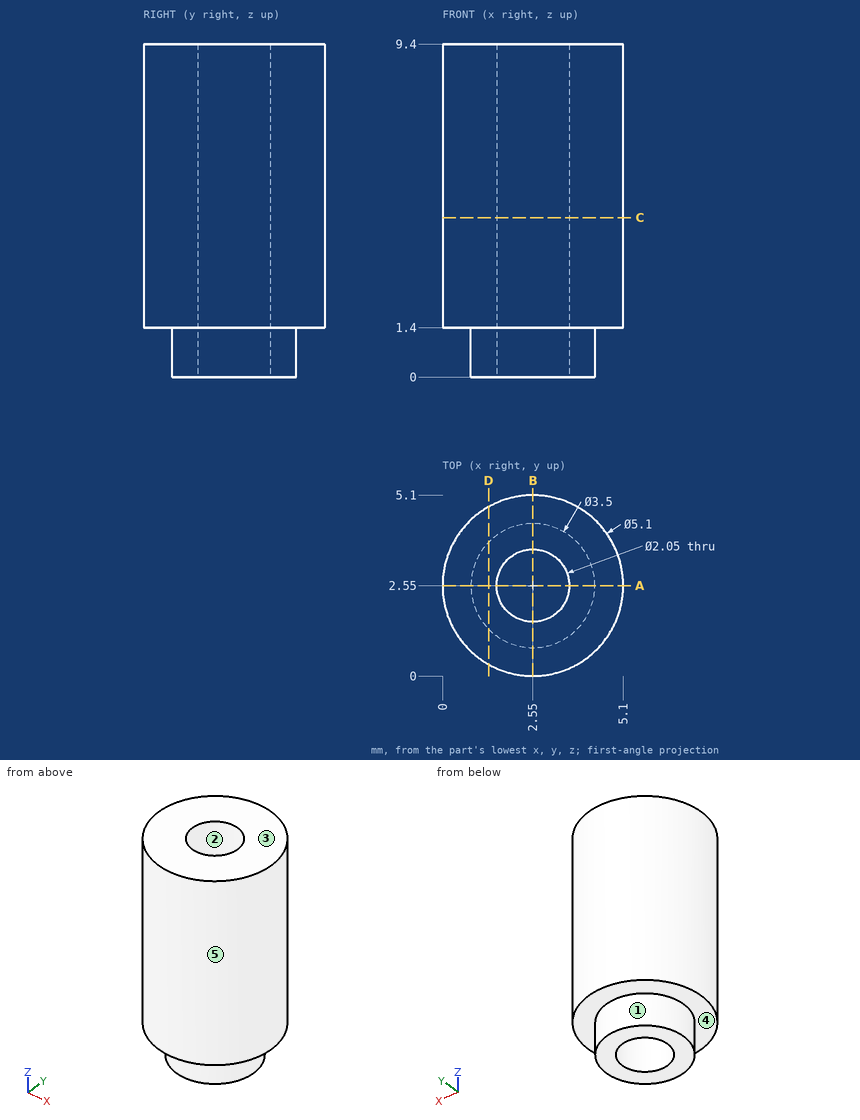
Print and shaded views of the part. All mm, measured from the part's lowest x, y and z. A direction names the side the tool comes from. Round coordinates to 2 decimals unless told otherwise and drop trailing zeros. Loops run counter-clockwise (first coordinate to the right, second up) from the corner with the lowest first, then second, coordinate; pieces in that order, holes last. Notation, with made-up numbers: (18, 30.25) -> (50, 30.25) arc R9 cw to (50, 41.25) -> close; hole circle Ø10 at (-16, 7). An arc over 180 degrees is marked (long way). Use CSV: the item, a comma, the result in double quotes. Start each with the question number.
1) Which spindle directions (+Z, -Z, +X, -X, +Y, -Y) get a long thin tool onto all of the face, cutting with end or side? Do the marked faces 4 and 5. Say none if no direction does.
2) Cut at A-A, the plane y = 2.55. Write the cut outline in (x, z) (3 decimals).
3) Pull direction Y, two halves, no side cores. Call the marked faces 1, 2 and 3: +Y half, -Y half, draft (parallel to the pull), parting line (faces both ways), or undercut.
4) Cut at D-D, the plane x = 1.3. Write the cut outline in (y, z).
5) Drop flat-ended pins along their axis: P1, Ø2, axis at y = 3.5, z = 5.5, coming from the +X side; P2, Ø1, axis at y = 4.5, z = 5, coming from the -X side. Give the stop position or say it passes through.
6) Cut at C-C, the plane z = 4.5. Write the cut outline in (x, y) (3 decimals), plus the area to 3 significant figures.
7) Wall check: L1, parallel to Y at x = 2.55, z = 2.5 (3 decimals); L2, parallel to Z at x = 0.8, y = 1.7; L3, parallel to Y at x = 3, z = 3.75. Give the ranges that are in metal, low to high. Write a range as [from, to].
Determined:
1,face 4,"-Z"
1,face 5,"+Z, -Z"
2,outline,"(0, 1.4) -> (0.8, 1.4) -> (0.8, 0) -> (1.525, 0) -> (1.525, 9.4) -> (0, 9.4) -> close; (3.575, 0) -> (4.3, 0) -> (4.3, 1.4) -> (5.1, 1.4) -> (5.1, 9.4) -> (3.575, 9.4) -> close"
3,face 1,"parting line"
3,face 2,"undercut"
3,face 3,"draft"
4,outline,"(0.33, 1.4) -> (1.33, 1.4) -> (1.33, 0) -> (3.77, 0) -> (3.77, 1.4) -> (4.77, 1.4) -> (4.77, 9.4) -> (0.33, 9.4) -> close"
5,P1,"stops at x = 5.1"
5,P2,"stops at x = 0.45"
6,outline,"circle Ø5.1 at (2.55, 2.55); hole circle Ø2.05 at (2.55, 2.55)"
6,area,"17.1 mm2"
7,L1,"y = [0, 1.525], [3.575, 5.1]"
7,L2,"z = [1.4, 9.4]"
7,L3,"y = [0.04, 1.63], [3.47, 5.06]"
